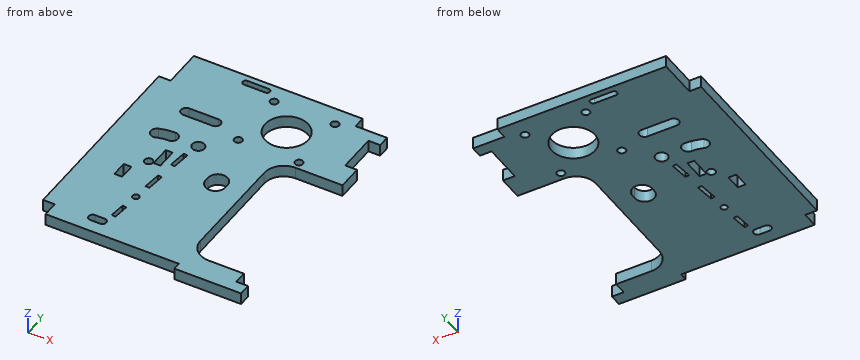
from build123d import *

# Parameters (mm, degrees)
ESQUISSE1_R        = 2
ESQUISSE1_R_2      = 11
ESQUISSE1_R_3      = 3.125
ESQUISSE1_R_4      = 2.1
ESQUISSE1_R_5      = 1.65
ESQUISSE1_W        = 4
ESQUISSE1_H        = 8
ESQUISSE1_W_2      = 3.5
ESQUISSE1_H_2      = 10.5
BOSS_EXTRU_1_DEPTH = 6


with BuildPart() as part:
    # Esquisse1 → Boss.-Extru.1 (new body)
    with BuildSketch(Plane.XY):
        with BuildLine():
            Line((2401.475943532, -52.104091931), (2401.475943532, -46.104091931))
            Line((2401.475943532, -46.104091931), (2395.475943532, -46.104091931))
            Line((2395.475943532, -46.104091931), (2395.475943532, -39.604091931))
            Line((2395.475943532, -39.604091931), (2377.475943532, -39.604091931))
            ThreePointArc((2377.475943532, -39.604091931), (2370.40487572, -36.675159743), (2367.475943532, -29.604091931))
            Line((2367.475943532, -29.604091931), (2367.475943532, 25.395908069))
            ThreePointArc((2367.475943532, 25.395908069), (2370.40487572, 32.466975881), (2377.475943532, 35.395908069))
            Line((2377.475943532, 35.395908069), (2397.475943532, 35.395908069))
            Line((2397.475943532, 35.395908069), (2401.475943532, 35.395908069))
            Line((2401.475943532, 35.395908069), (2401.475943532, 47.895908069))
            Line((2401.475943532, 47.895908069), (2395.475943532, 47.895908069))
            Line((2395.475943532, 47.895908069), (2395.475943532, 67.895908069))
            Line((2395.475943532, 67.895908069), (2401.475943532, 67.895908069))
            Line((2401.475943532, 67.895908069), (2401.475943532, 73.792808343))
            Line((2401.475943532, 73.792808343), (2395.475943532, 73.792808343))
            Line((2395.475943532, 73.792808343), (2385.475943532, 73.792808343))
            Line((2385.475943532, 73.792808343), (2385.475943532, 79.792808343))
            Line((2385.475943532, 79.792808343), (2299.475943532, 79.792808343))
            Line((2299.475943532, 79.792808343), (2299.475943532, 59.792808343))
            Line((2299.475943532, 59.792808343), (2293.475943532, 59.792808343))
            Line((2293.475943532, 59.792808343), (2293.475943532, -40.20719166))
            Line((2293.475943532, -40.20719166), (2299.475943532, -40.20719166))
            Line((2299.475943532, -40.20719166), (2299.475943532, -48.20719166))
            Line((2299.475943532, -48.20719166), (2367.475943532, -48.20719166))
            Line((2367.475943532, -48.20719166), (2367.475943532, -52.104091931))
            Line((2367.475943532, -52.104091931), (2401.475943532, -52.104091931))
        make_face()
        with Locations((2346.01021478, 70.349007801)):
            Circle(ESQUISSE1_R, mode=Mode.SUBTRACT)
        with Locations((2377.01021478, 70.349007801)):
            Circle(ESQUISSE1_R, mode=Mode.SUBTRACT)
        with Locations((2377.01021478, 39.349007801)):
            Circle(ESQUISSE1_R, mode=Mode.SUBTRACT)
        with Locations((2361.51021478, 54.849007801)):
            Circle(ESQUISSE1_R_2, mode=Mode.SUBTRACT)
        with Locations((2346.01021478, 39.349007801)):
            Circle(ESQUISSE1_R, mode=Mode.SUBTRACT)
        with Locations((2333.225943532, 26.564736553)):
            Circle(ESQUISSE1_R_3, mode=Mode.SUBTRACT)
        with Locations((2319.725943533, 6.564736553)):
            Circle(ESQUISSE1_R_4, mode=Mode.SUBTRACT)
        with Locations((2327.476078896, -17.594891177)):
            Circle(ESQUISSE1_R_5, mode=Mode.SUBTRACT)
        with BuildLine():
            Line((2331.275943532, 42.100855433), (2316.275943532, 42.100855433))
            ThreePointArc((2316.275943532, 42.100855433), (2313.675943532, 44.700855433), (2316.275943532, 47.300855433))
            Line((2316.275943532, 47.300855433), (2331.275943532, 47.300855433))
            ThreePointArc((2331.275943532, 47.300855433), (2333.875943532, 44.700855433), (2331.275943532, 42.100855433))
        make_face(mode=Mode.SUBTRACT)
        with BuildLine():
            Line((2347.975943532, 7.895908069), (2347.975943532, 9.895908069))
            ThreePointArc((2347.975943532, 9.895908069), (2352.975943532, 14.895908069), (2357.975943532, 9.895908069))
            Line((2357.975943532, 9.895908069), (2357.975943532, 7.895908069))
            ThreePointArc((2357.975943532, 7.895908069), (2352.975943532, 2.895908069), (2347.975943532, 7.895908069))
        make_face(mode=Mode.SUBTRACT)
        with BuildLine():
            Line((2339.47303261, 73.792808343), (2328.599494457, 73.792808343))
            ThreePointArc((2328.599494457, 73.792808343), (2327.099494457, 75.292808343), (2328.599494457, 76.792808343))
            Line((2328.599494457, 76.792808343), (2339.47303261, 76.792808343))
            ThreePointArc((2339.47303261, 76.792808343), (2340.97303261, 75.292808343), (2339.47303261, 73.792808343))
        make_face(mode=Mode.SUBTRACT)
        with Locations((2313.225943533, -4.641462904)):
            Rectangle(ESQUISSE1_W, ESQUISSE1_H, mode=Mode.SUBTRACT)
        Polygon((2329.302925864, 9.55284837), (2330.275943532, 18.879356423), (2332.265147216, 18.67182641), (2331.292129548, 9.345318358), align=None, mode=Mode.SUBTRACT)
        Polygon((2327.356890528, -9.100167734), (2328.329908196, 0.226340318), (2330.31911188, 0.018810306), (2329.346094212, -9.307697746), align=None, mode=Mode.SUBTRACT)
        Polygon((2324.775943532, -33.838899342), (2325.606063581, -25.882084609), (2327.595267264, -26.089614621), (2326.765147216, -34.046429354), align=None, mode=Mode.SUBTRACT)
        with Locations((2323.975943533, 11.814736553)):
            Rectangle(ESQUISSE1_W_2, ESQUISSE1_H_2, mode=Mode.SUBTRACT)
        with BuildLine():
            Line((2318.475943532, -37.70719166), (2323.475943532, -37.70719166))
            ThreePointArc((2323.475943532, -37.70719166), (2325.475943532, -39.70719166), (2323.475943532, -41.70719166))
            Line((2323.475943532, -41.70719166), (2318.475943532, -41.70719166))
            ThreePointArc((2318.475943532, -41.70719166), (2316.475943532, -39.70719166), (2318.475943532, -37.70719166))
        make_face(mode=Mode.SUBTRACT)
        with BuildLine():
            ThreePointArc((2319.725943533, 29.694736553), (2315.709461183, 29.34333988), (2311.815017618, 28.299826872))
            ThreePointArc((2311.815017618, 28.299826872), (2309.944302763, 24.28806592), (2313.956063715, 22.417351066))
            ThreePointArc((2313.956063715, 22.417351066), (2316.796498776, 23.178443347), (2319.725943533, 23.434736553))
            ThreePointArc((2319.725943533, 23.434736553), (2322.855943533, 26.564736553), (2319.725943533, 29.694736553))
        make_face(mode=Mode.SUBTRACT)
    extrude(amount=-BOSS_EXTRU_1_DEPTH)


solid = part.part
The model under review builds one solid part; all positions refer to its coordinate system, in mm. Coordinates: 2 decimals unless noted, no trailing zeros. Order: outer loops, then holes, each group sorted by start corner. A loop starts at its lowest first (then second) coordinate and runs counter-clockwise, first axis right, second up. Notation, with made-up numbers: (29, -1) -> (82, -1) arc R35 cw to (82, 38) -> close; hole circle Ø9 at (2, 71.25). An arc over 180 degrees is marked (long way). Answer in a Markdown table with one row per item.
(1) Consider section C-C (z = -2.75). State how many separate pieces and enclosed holes the cut face has, plus the area to 3 significant figures.
Answers:
| item | result |
|---|---|
| separate pieces | 1 |
| enclosed holes | 18 |
| area | 10,100 mm² |
(2) Consider section D-D (y = -14). Write out the cut boundary in (x, z).
Answers:
| item | result |
|---|---|
| outline | (2293.48, -6) -> (2367.48, -6) -> (2367.48, 0) -> (2293.48, 0) -> close |
(3) Wall thickness on line 1 along X through (y, z) = (39.5, -0.9); line 2 along X through (y, z) = (55.5, -1.85); line 3 along Y through (x, z) = (2345.5, -3.6): over which ranges is each line inside the solid? List them lowest first.
Answers:
| item | result |
|---|---|
| line 1 | 2293.48 to 2344.02, 2348 to 2375.02, 2379 to 2401.48 |
| line 2 | 2293.48 to 2350.53, 2372.49 to 2395.48 |
| line 3 | -48.21 to 37.42, 41.28 to 68.42, 72.28 to 79.79 |
(4) Insertion check: pin 1 (6 mm diameter, centred on x = 2373.5, y = -34, fed in from -Z); pin 2 (1.6 mm diameter, centred on y = 8.5, z = -3.5, fed in from +X); pin 3 (3 mm diameter, centred on x = 2309, z = -3, fed in from -Y); pin 4 (1.8 mm diameter, centred on x = 2399.5, z = -4.5, fed in from +Y). Each pin has a flat end and moves straight along its axis. Give the tip position at first contact, or say it passes through.
Answers:
| item | result |
|---|---|
| pin 1 | through |
| pin 2 | x = 2367.48 |
| pin 3 | y = -48.21 |
| pin 4 | y = 73.79 |
(5) Consider section A-A (x = 2362). Write out the cut boundary in (y, z), plus the area to 3 significant figures.
Answers:
| item | result |
|---|---|
| outline | (-48.21, -6) -> (43.86, -6) -> (43.86, 0) -> (-48.21, 0) -> close; (65.84, -6) -> (79.79, -6) -> (79.79, 0) -> (65.84, 0) -> close |
| area | 636 mm² |
(6) Consider section B-B (y = -31). Write out the cut boundary in (x, z), plus the area to 3 significant figures.
Answers:
| item | result |
|---|---|
| outline | (2293.48, -6) -> (2325.07, -6) -> (2325.07, 0) -> (2293.48, 0) -> close; (2327.08, -6) -> (2367.57, -6) -> (2367.57, 0) -> (2327.08, 0) -> close |
| area | 433 mm² |
